```python
from build123d import *

# Parameters (mm, degrees)
F0_W      = 280
F0_H      = 280
F0_W_2    = 50
F0_H_2    = 50
F1_DEPTH  = 18
F2_DEPTH  = 2
F3_W      = 16
F3_H      = 6
F4_DEPTH  = 115
F5_W      = 280
F5_H      = 280
F5_W_2    = 50
F5_H_2    = 50
F5_W_3    = 16
F5_H_3    = 16
F6_DEPTH  = 2
F7_W      = 26
F7_H      = 26
F7_W_2    = 18
F7_H_2    = 18
F8_DEPTH  = 4
F10_D     = 2.7
F10_DEPTH = 8
F10_TIP   = 0.8111618357
F9_W      = 5
F9_H      = 4
F11_DEPTH = 4


with BuildPart() as f1:
    # F0 (on Top) → F1 (new body)
    with BuildSketch(Plane.XY):
        Rectangle(F0_W, F0_H)
        Rectangle(F0_W_2, F0_H_2, mode=Mode.SUBTRACT)
    extrude(amount=F1_DEPTH)

    # F0 (on Top) → F2 (join)
    with BuildSketch(Plane.XY):
        Rectangle(F0_W, F0_H)
        Rectangle(F0_W_2, F0_H_2, mode=Mode.SUBTRACT)
        Rectangle(F0_W_2, F0_H_2)
    extrude(amount=-F2_DEPTH)

    # F3 (on face) → F4 (cut, through all)
    with BuildSketch(Plane.YZ.offset(140)):
        with Locations((0.0201961273, 3)):
            Rectangle(F3_W, F3_H)
    extrude(amount=-F4_DEPTH, mode=Mode.SUBTRACT)


with BuildPart() as f6:
    # F5 (on face) → F6 (new body)
    with BuildSketch(Plane.XY.offset(18)):
        Rectangle(F5_W, F5_H)
        Rectangle(F5_W_2, F5_H_2, mode=Mode.SUBTRACT)
        Rectangle(F5_W_2, F5_H_2)
        Rectangle(F5_W_3, F5_H_3, mode=Mode.SUBTRACT)
    extrude(amount=F6_DEPTH)

    # F7 (on face) → F8 (join)
    with BuildSketch(Plane.XY.offset(20)):
        Rectangle(F7_W, F7_H)
        Rectangle(F7_W_2, F7_H_2, mode=Mode.SUBTRACT)
    extrude(amount=F8_DEPTH)

    # F10
    with Locations(Plane.XY.offset(24)):
        with Locations((-10.5, 10.5), (10.5, 10.5), (-10.5, -10.5), (10.5, -10.5)):
            Hole(F10_D / 2, depth=F10_DEPTH)
            with Locations((0, 0, -(F10_DEPTH + F10_TIP / 2))):  # 118° drill point
                Cone(0, F10_D / 2, F10_TIP, mode=Mode.SUBTRACT)

    # F9 (on face) → F11 (cut, through all)
    with BuildSketch(Plane.XY.offset(24)):
        with Locations((0, 11)):
            Rectangle(F9_W, F9_H)
        with Locations((0, -11)):
            Rectangle(F9_W, F9_H)
    extrude(amount=-F11_DEPTH, mode=Mode.SUBTRACT)


solid = f6.part
```
Verification items for the finished model (mm, model axes). Give positions to 0.01 mm unless a question says otherwise; leave off trailing zeros. Order: outer loops, then holes, each group sorted by start corner. A loop starts at its lowest first (then second) coordinate and runs counter-clockwise, first axis right, second up. Notation, with made-up numbers: (-22.75, 3) -> (23.25, 3) arc R4 ccw to (23.25, 8) -> close; hole circle Ø8 at (37, 88.5). An arc over 180 degrees is marked (long way). Use a Markdown table: item, result.
1) Section check B-B, the plane x = -118. Record the boundary of the cut face in (y, z).
Results:
| item | result |
|---|---|
| outline | (-140, 18) -> (140, 18) -> (140, 20) -> (-140, 20) -> close |
2) Material ranges on probe 1 along Y at (x, z) = (10.5, 22.8); probe 2 along Y at (x, z) = (-10.5, 19.45); probe 3 along Z at (x, y) = (87.5, 56), recorded low to high.
Results:
| item | result |
|---|---|
| probe 1 | -13 to -11.85, -9.15 to 9.15, 11.85 to 13 |
| probe 2 | -140 to -11.85, -9.15 to 9.15, 11.85 to 140 |
| probe 3 | 18 to 20 |
3) Depth check by flat-ended pin: pin 1 Ø1.2 at (x, z) = (5.5, 21.5) entering from +Y; pin 2 Ø1.5 at (x, y) = (-84.5, 75) entering from +Z; pin 3 Ø3 at (x, z) = (7, 22.5) entering from -Y; pin 4 Ø2.5 at (x, y) = (-10.5, -10.5) entering from -Z. Enter the tip coordinate at first touch or a pass-through.
Results:
| item | result |
|---|---|
| pin 1 | y = 13 |
| pin 2 | z = 20 |
| pin 3 | y = -13 |
| pin 4 | through |
4) Section check A-A, the plane z = 22.8. Record the boundary of the cut face in (x, y), then the cut area to 3 significant figures.
Results:
| item | result |
|---|---|
| outline | (-13, -13) -> (-2.5, -13) -> (-2.5, -9) -> (-9, -9) -> (-9, 9) -> (-2.5, 9) -> (-2.5, 13) -> (-13, 13) -> close; (2.5, -13) -> (13, -13) -> (13, 13) -> (2.5, 13) -> (2.5, 9) -> (9, 9) -> (9, -9) -> (2.5, -9) -> close; hole circle Ø2.7 at (-10.5, -10.5); hole circle Ø2.7 at (-10.5, 10.5); hole circle Ø2.7 at (10.5, -10.5); hole circle Ø2.7 at (10.5, 10.5) |
| area | 289 mm² |
